Read the model definition and answer for the solid it produces. Units are mm, in the model's axes. Coordinates: 2 decimals unless noted, no trailing zeros. Write each loop counter-clockwise with the first axis right and the second up, starting at its lowest first coordinate (ties: lowest second). Pieces come first, ordered by that corner, then holes.
(1) Section A-A on y = 15 is taken. Write down the section's boundary in (x, z).
(2) Section B-B on x = 0 is taken. Write down the section's boundary in (y, z).
(3) Section C-C on z = 2.5 is taken. Write down the section's boundary in (x, y), then the cut area to 3 significant figures.
(4) Find the intervals of material crossed by probe 1 along Y at (x, z) = (0, -0.2); probe 2 along X at (y, z) = (14, -1.25), in increasing order.
Autodesk Inventor part; units mm, degrees
sketch "Sketch1" plane through (0, 0, 0) normal (0, 0, 1) x (1, 0, 0)
  line L0 (-50, 25) -> (50, 25)
  line L1 (50, 25) -> (50, -25)
  line L2 (50, -25) -> (-50, -25)
  line L3 (-50, -25) -> (-50, 25)
  line L4 (-50, 25) -> (50, -25) construction
  line L5 (50, 25) -> (-50, -25) construction
  circle A0 centre (0, 15) radius 5.2
  circle A1 centre (0, 15) radius 5
  point P0 (0, 0)
  point P1 (0, 0)
  dimension "d0" = 100
  dimension "d1" = 50
  dimension "d2" = 15
  dimension "d7" = 10.4
extrude "Extrusion1" add sketch "Sketch1" along normal mid plane 7 contours L0 L1 L2 L3
fillet "Fillet1" radius 5 2 edges at (50, 25, 0) (-50, 25, 0)
chamfer "Chamfer1" distance 2 angle 45 1 edges at (-5.2, 15, 3.5)
properties part number "sessao_07_04_003_001"
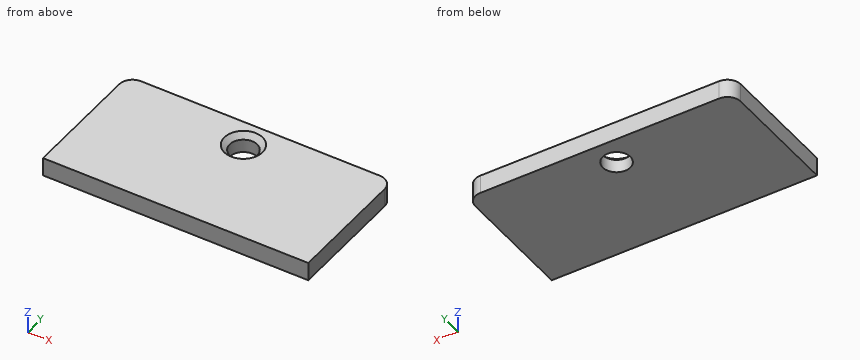
Response:
1. outline: (-50, -3.5) - (-5.2, -3.5) - (-5.2, 1.5) - (-7.2, 3.5) - (-50, 3.5) - close; (5.2, -3.5) - (50, -3.5) - (50, 3.5) - (7.2, 3.5) - (5.2, 1.5) - close
2. outline: (-25, -3.5) - (9.8, -3.5) - (9.8, 1.5) - (7.8, 3.5) - (-25, 3.5) - close; (20.2, -3.5) - (25, -3.5) - (25, 3.5) - (22.2, 3.5) - (20.2, 1.5) - close
3. outline: (-50, -25) - (50, -25) - (50, 20) arc R5 ccw to (45, 25) - (-45, 25) arc R5 ccw to (-50, 20) - close; hole circle Ø12.4 at (0, 15)
3. area: 4,870 mm2
4. probe 1: y = -25 to 9.8, 20.2 to 25
4. probe 2: x = -50 to -5.1, 5.1 to 50
